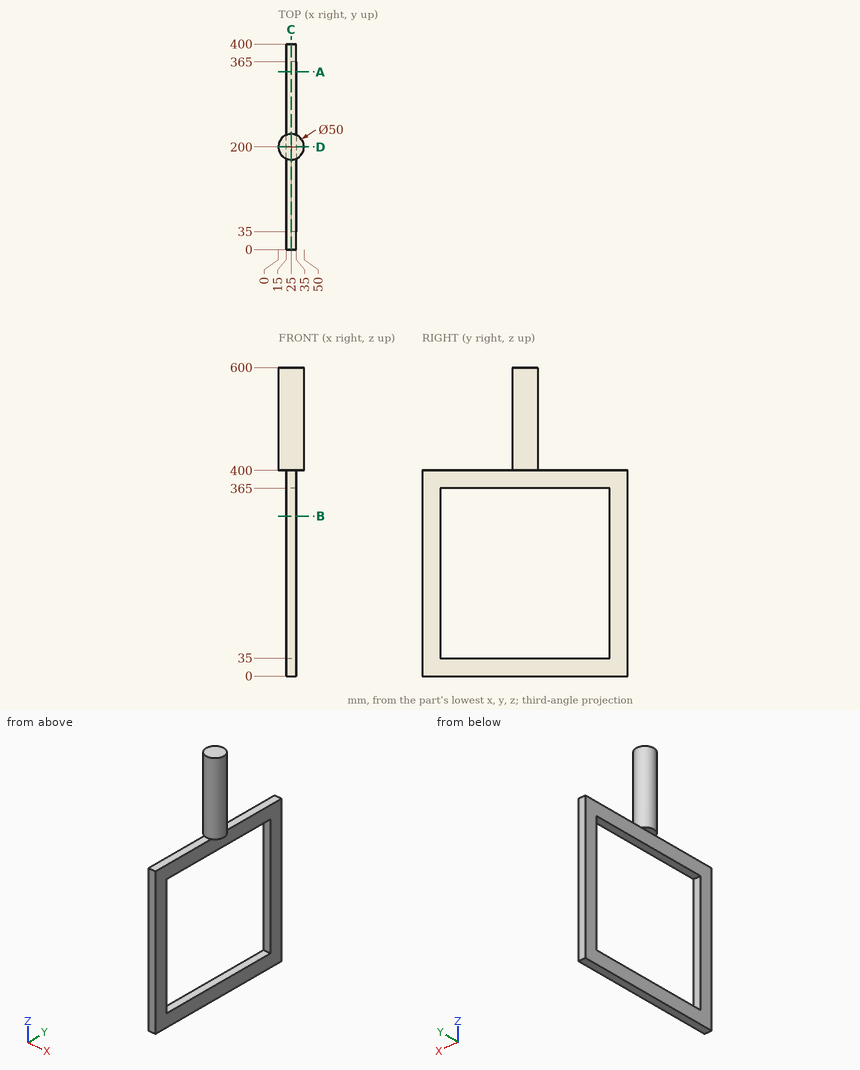
The figure shows three views and two pictorial views of one solid part (mm, origin at its lowest corner). Answer the questions. Coordinates: 2 decimals unless noted, no trailing zeros. Loops run counter-clockwise (first coordinate to the right, second up) from the corner with the lowest first, then second, coordinate; pieces in that order, holes last. Notation, with made-up numbers: (-10, 60.5) - (12, 60.5) arc R28 ccw to (12, 87.5) - close; hole circle Ø3 at (28.25, 39.5). An arc over 180 degrees is marked (long way). Use a Markdown table: item, result. Add a question column.
1) The part is cut by section C-C, the plane x = 25. Give the vertices of the cut face in (y, z), and give its area (3 significant figures).
2) Find the intervals of material crossed by line 1 (Z direction, x = 23, y = 153.5); line 2 (X direction, y = 373.5, z = 225.5), in increasing order.
3) The part is cut by section A-A, the plane y = 346. Give the vertices of the cut face in (x, z).
4) Given pin 1 (12 mm diameter, centred on x = 12.5, z = 497, fed in from -Y); pin 2 (10 mm diameter, centred on x = 27.5, y = 60, fed in from -Z); pin 3 (6 mm diameter, centred on x = 23, y = 126, fed in from +Z); pin 4 (7.5 mm diameter, centred on x = 10.5, y = 210.5, fed in from -Z), each flat-ended and moving along its own axis, determine where each tip first touches the part or whether it passes through.
5) The part is cut by section D-D, the plane y = 200. Give the vertices of the cut face in (x, z), and give its area (3 significant figures).
Here are the results:
| question | item | result |
|---|---|---|
| 1 | outline | (0, 0) - (400, 0) - (400, 400) - (225, 400) - (225, 600) - (175, 600) - (175, 400) - (0, 400) - close; hole (35, 35) - (365, 35) - (365, 365) - (35, 365) - close |
| 1 | area | 61,100 mm^2 |
| 2 | line 1 | z = 0 to 35, 365 to 400 |
| 2 | line 2 | x = 15 to 35 |
| 3 | outline | (15, 0) - (35, 0) - (35, 35) - (15, 35) - close; (15, 365) - (35, 365) - (35, 400) - (15, 400) - close |
| 4 | pin 1 | stops at y = 175.86 |
| 4 | pin 2 | stops at z = 0 |
| 4 | pin 3 | stops at z = 400 |
| 4 | pin 4 | stops at z = 400 |
| 5 | outline | (0, 400) - (15, 400) - (15, 365) - (35, 365) - (35, 400) - (50, 400) - (50, 600) - (0, 600) - close; (15, 0) - (35, 0) - (35, 35) - (15, 35) - close |
| 5 | area | 11,400 mm^2 |
